Could you check a few things on this model? Use its own coordinates, in mm. Face numbers are marked on the shaded views. A direction names the side the tool comes from. Round coordinates to 2 decimals unless told otherwise and drop trailing zeros. Write each loop counter-clockwise with the first axis right and the second up, starting at its lowest first coordinate (ties: lowest second). Pieces come first, ordered by that corner, then holes. Notation, with made-up numbers: (-0.5, -21.75) -> (25.5, -21.75) arc R14 ccw to (25.5, -6.75) -> close; hole circle Ø1 at (-1.5, 34). An arc over 180 degrees is marked (long way). One line per question, with ' | ' between items. Start each with the question number.
1. Imagine slicing it at A-A, the plane y = -67. List the corners of the cut face in (x, z) for me (3 decimals).
2. If I drill on line 1 along X through (y, z) = (39.5, -41.5); line 2 along Y through (x, z) = (3.25, 24), over which ranges is the centre line in solid material (lowest first)? Write a range as [from, to].
3. Imagine slicing it at B-B, the plane x = -7.75. List the corners of the cut face in (y, z) for me.
4. Imagine slicing it at C-C, the plane z = 31. List the corners of the cut face in (x, y) for me.
5. Imagine slicing it at D-D, the plane y = 5. List the corners of the cut face in (x, z) for me.
6. For pin 1 Ø4.5 at (x, z) = (-8.5, 28.5) entering from -Y; pin 2 Ø8 at (x, y) = (-6, 60) entering from +Z; pin 3 Ø4.5 at (x, y) = (-4, -11) entering from +Z; pin 4 Ø1 at (y, z) = (33, -9) entering from -X, each with a flat end and sliding along its axis, tell me the tip position at first contact or that it passes through.
7. For the marked faces 1, 2, 3 and 4, which set-ups out of +Z, -Z, +X, -X, +Y, -Y let a thin tool reach every point of the face, with its end or its side?
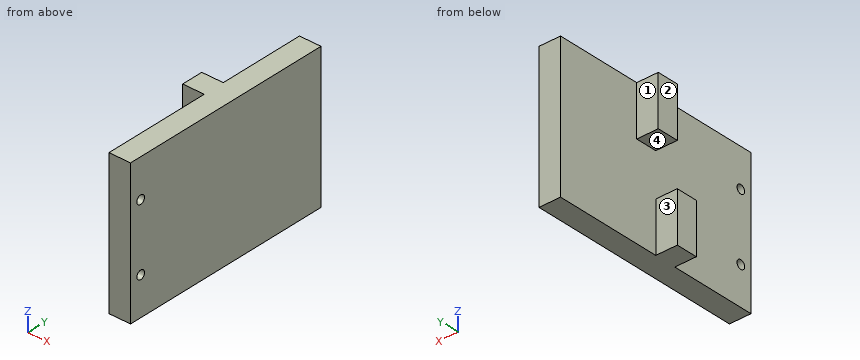
from build123d import *

# Parameters (mm, degrees)
CROQUIS1_W              = 100
CROQUIS1_H              = 150
SALIENTE_EXTRUIR1_DEPTH = 15
CROQUIS2_W              = 35
CROQUIS2_H              = 15
SALIENTE_EXTRUIR2_DEPTH = 15
CROQUIS3_R              = 3
CORTAR_EXTRUIR1_DEPTH   = 96


with BuildPart() as part:
    # Croquis1 → Saliente-Extruir1 (new body)
    with BuildSketch(Plane(origin=(0, 0, 0), x_dir=(0, 0, -1), z_dir=(1, 0, 0))):
        Rectangle(CROQUIS1_W, CROQUIS1_H)
    extrude(amount=SALIENTE_EXTRUIR1_DEPTH)

    # Croquis2 → Saliente-Extruir2 (add)
    with BuildSketch(Plane.ZY):
        with Locations((32.5, 7.5)):
            Rectangle(CROQUIS2_W, CROQUIS2_H)
        with Locations((-32.5, -7.5)):
            Rectangle(CROQUIS2_W, CROQUIS2_H)
    extrude(amount=SALIENTE_EXTRUIR2_DEPTH)

    # Croquis3 → Cortar-Extruir1 (cut, through all)
    with BuildSketch(Plane(origin=(15, 0, 0), x_dir=(0, 0, -1), z_dir=(1, 0, 0))):
        with Locations((-23.345, -67)):
            Circle(CROQUIS3_R)
        with Locations((23.345, -67)):
            Circle(CROQUIS3_R)
    extrude(amount=-CORTAR_EXTRUIR1_DEPTH, mode=Mode.SUBTRACT)


solid = part.part
Geometry results:
1) outline: (0, -50) -> (15, -50) -> (15, -26.345) -> (0, -26.345) -> close; (0, -20.345) -> (15, -20.345) -> (15, 20.345) -> (0, 20.345) -> close; (0, 26.345) -> (15, 26.345) -> (15, 50) -> (0, 50) -> close
2) line 1: x = [0, 15] | line 2: y = [-75, -69.93], [-64.07, 75]
3) outline: (-15, -50) -> (0, -50) -> (0, -15) -> (-15, -15) -> close; (0, 15) -> (15, 15) -> (15, 50) -> (0, 50) -> close
4) outline: (-15, 0) -> (0, 0) -> (0, -75) -> (15, -75) -> (15, 75) -> (0, 75) -> (0, 15) -> (-15, 15) -> close
5) outline: (-15, 15) -> (0, 15) -> (0, -50) -> (15, -50) -> (15, 50) -> (-15, 50) -> close
6) pin 1: stops at y = 0 | pin 2: passes through | pin 3: stops at z = -15 | pin 4: stops at x = 0
7) face 1: +Z, -Z, -X, +Y | face 2: +Z, -Z, -X, +Y, -Y | face 3: -Z, -X, +Y | face 4: -Z, -X, +Y, -Y
